from build123d import *

# Parameters (mm, degrees)
SKETCH2_W          = 47.8
SKETCH2_H          = 3.8575
CHAMFER1_SIZE      = 1.5
CHAMFER2_SIZE      = 0.5
SKETCH3_R          = 3
CUT_EXTRUDE1_DEPTH = 56.546738091


with BuildPart() as part:
    # Sketch2 → Revolve1 (revolve)
    with BuildSketch(Plane.XY, mode=Mode.PRIVATE) as revolve1_sk:
        with Locations((-23.9, 18.07875)):
            Rectangle(SKETCH2_W, SKETCH2_H)
    revolve(revolve1_sk.sketch.rotate(Axis((0, 0, 0), (-1, 0, 0)), 90), axis=Axis((0, 0, 0), (-1, 0, 0)))

    # Chamfer1
    chamfer1_edges = [part.edges().sort_by_distance(p)[0] for p in [
        (-47.8, 0, 20.0075),
        (0, 0, 20.0075),
    ]]
    chamfer(chamfer1_edges, length=CHAMFER1_SIZE)

    # Chamfer2
    chamfer2_edges = [part.edges().sort_by_distance(p)[0] for p in [
        (-47.8, 0, 16.15),
        (0, 0, 16.15),
    ]]
    chamfer(chamfer2_edges, length=CHAMFER2_SIZE)

    # Sketch3 → Cut-Extrude1 (cut, through all)
    with BuildSketch(Plane(origin=(0, 0, 0), x_dir=(1, 0, 0), z_dir=(0, 1, 0))):
        with Locations(Location((-16, 0, 0), (0, 0, 270))):
            Circle(SKETCH3_R)
        with Locations(Location((-32, 0, 0), (0, 0, 270))):
            Circle(SKETCH3_R)
    extrude(amount=-CUT_EXTRUDE1_DEPTH, mode=Mode.SUBTRACT)


solid = part.part
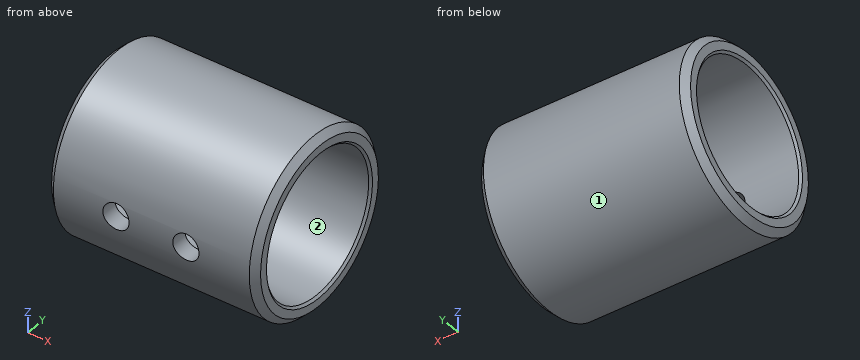
Verification items for the finished model (mm, model axes). Face numbers are marked on the shaded views. Coordinates: 2 decimals unless noted, no trailing zeros. Write each loop counter-clockwise with the first axis right and the second up, starting at its lowest first coordinate (ties: lowest second). Pieces come first, ordered by that corner, then holes. Notation, with made-up numbers: M -14,42.5 L -7,42.5 A16 ccw -7,49.5 Z; hole C 75.5,68.25 d10. An arc over 180 degrees is marked long. Use CSV: the item, a comma, the result in double quotes.
Q1. Thickness scan on line 1 along X through (y, z) = (-18, 0); line 2 along X through (y, z) = (-18.95, 0); line 3 along Z through (x, y) = (-16, -18) (3 decimals). Record the ranges inside material, lowest first. Write a range as [from, to].
Computed values:
line 1,"[-47.8, -35], [-29, -19], [-13, 0]"
line 2,"[-47.36, -35], [-29, -19], [-13, -0.44]"
line 3,"[-8.735, -3], [3, 8.735]"
Q2. Mould release check, pull along Y, two halves, no side actions. Record for the marked faces 1 and 2: pulls with the +Y half, pulls with the -Y half, needs draft (parallel to the pull), parting line crosses it, or undercut.
Computed values:
face 1,"parting line crosses it"
face 2,"undercut"
Q3. Section check B-B, the plane y = 0. Enter the section's corners in (x, z).
Computed values:
outline,"M -47.8,-18.51 L -46.3,-20.01 L -1.5,-20.01 L 0,-18.51 L 0,-16.65 L -0.5,-16.15 L -47.3,-16.15 L -47.8,-16.65 Z; M -47.8,16.65 L -47.3,16.15 L -0.5,16.15 L 0,16.65 L 0,18.51 L -1.5,20.01 L -46.3,20.01 L -47.8,18.51 Z"
Q4. Section check A-A, the plane z = 0. Enter the section's corners in (x, y), and give its area (3 significant figures).
Computed values:
outline,"M -47.8,-18.51 L -46.3,-20.01 L -35,-20.01 L -35,-16.15 L -47.3,-16.15 L -47.8,-16.65 Z; M -47.8,16.65 L -47.3,16.15 L -0.5,16.15 L 0,16.65 L 0,18.51 L -1.5,20.01 L -46.3,20.01 L -47.8,18.51 Z; M -29,-20.01 L -19,-20.01 L -19,-16.15 L -29,-16.15 Z; M -13,-20.01 L -1.5,-20.01 L 0,-18.51 L 0,-16.65 L -0.5,-16.15 L -13,-16.15 Z"
area,"317 mm²"
Q5. Go/stop test with flat-tipped pins: P1, Ø2, axis at x = -39, y = 3.5, coming from the +Z side; P2, Ø4, axis at x = -20, y = -14, coming from the +Z side; P3, Ø4, axis at x = -20, z = -11, coming from the -Y side. Record where each tip stops, or that it passes through.
Computed values:
P1,"z = 19.85"
P2,"z = 16.01"
P3,"y = -17.87"
